from build123d import *

# Parameters (mm, degrees)
SKETCH1_W                = 25
SKETCH1_H                = 120.5
SKETCH1_H_2              = 25
BOSS_EXTRUDE1_DEPTH      = 25
SKETCH1_8_W              = 25
SKETCH1_8_H              = 25
BOSS_EXTRUDE2_DEPTH      = 90
SKETCH1_9_W              = 25
SKETCH1_9_H              = 25
BOSS_EXTRUDE3_DEPTH      = 90
BOSS_EXTRUDE3_DEPTH_BACK = 130
BOSS_EXTRUDE4_DEPTH      = 75
BOSS_EXTRUDE4_DEPTH_BACK = 100
SKETCH3_R                = 16
SKETCH3_R_2              = 12.5
BOSS_EXTRUDE5_DEPTH      = 2
BOSS_EXTRUDE5_DEPTH_BACK = 2
SKETCH4_R                = 16
BOSS_EXTRUDE6_DEPTH      = 2
BOSS_EXTRUDE6_DEPTH_BACK = 2


with BuildPart() as part:
    # Sketch1 → Boss-Extrude1 (new body)
    with BuildSketch(Plane(origin=(0, 0, 0), x_dir=(1, 0, 0), z_dir=(0, 1, 0))):
        with Locations((-72.566666667, -14.316666667)):
            Rectangle(SKETCH1_W, SKETCH1_H)
        with Locations((-72.566666667, 58.433333333)):
            Rectangle(SKETCH1_W, SKETCH1_H_2)
        with Locations((-72.566666667, -87.066666667)):
            Rectangle(SKETCH1_W, SKETCH1_H_2)
    extrude(amount=BOSS_EXTRUDE1_DEPTH)

    # Sketch1_8 → Boss-Extrude2 (add)
    with BuildSketch(Plane(origin=(0, 0, 0), x_dir=(1, 0, 0), z_dir=(0, 1, 0))):
        with Locations((-72.566666667, 58.433333333)):
            Rectangle(SKETCH1_8_W, SKETCH1_8_H)
        with Locations((-72.566666667, -87.066666667)):
            Rectangle(SKETCH1_8_W, SKETCH1_8_H)
    extrude(amount=BOSS_EXTRUDE2_DEPTH)

    # Sketch1_9 → Boss-Extrude3 (add, two sides)
    with BuildSketch(Plane(origin=(0, 0, 0), x_dir=(1, 0, 0), z_dir=(0, 1, 0))) as boss_extrude3_sk:
        with Locations((-72.566666667, -87.066666667)):
            Rectangle(SKETCH1_9_W, SKETCH1_9_H)
    extrude(amount=BOSS_EXTRUDE3_DEPTH)
    extrude(boss_extrude3_sk.sketch, amount=-BOSS_EXTRUDE3_DEPTH_BACK)

    # Sketch2 → Boss-Extrude4 (add, two sides)
    with BuildSketch(Plane(origin=(-60.066666667, 0, 0), x_dir=(0, 0, -1), z_dir=(1, 0, 0))) as boss_extrude4_sk:
        with BuildLine():
            ThreePointArc((-99.566666667, -117.5), (-95.905501431, -126.338834765), (-87.066666667, -130))
            ThreePointArc((-87.066666667, -130), (-82.283123762, -129.048494156), (-78.227831902, -126.338834765))
            Line((-78.227831902, -126.338834765), (-95.905501431, -108.661165235))
            ThreePointArc((-95.905501431, -108.661165235), (-98.615160823, -112.716457095), (-99.566666667, -117.5))
        make_face()
        with BuildLine():
            Line((-95.905501431, -108.661165235), (-78.227831902, -126.338834765))
            ThreePointArc((-78.227831902, -126.338834765), (-75.51817251, -122.283542905), (-74.566666667, -117.5))
            ThreePointArc((-74.566666667, -117.5), (-78.227831902, -108.661165235), (-87.066666667, -105))
            ThreePointArc((-87.066666667, -105), (-91.850209571, -105.951505844), (-95.905501431, -108.661165235))
        make_face()
    extrude(amount=BOSS_EXTRUDE4_DEPTH)
    extrude(boss_extrude4_sk.sketch, amount=-BOSS_EXTRUDE4_DEPTH_BACK)

    # Sketch3 → Boss-Extrude5 (add, two sides)
    with BuildSketch(Plane(origin=(14.933333333, 0, 0), x_dir=(0, 0, -1), z_dir=(1, 0, 0))) as boss_extrude5_sk:
        with Locations((-87.066666667, -117.5)):
            Circle(SKETCH3_R)
        with Locations((-87.066666667, -117.5)):
            Circle(SKETCH3_R_2, mode=Mode.SUBTRACT)
        with BuildLine():
            ThreePointArc((-74.566666667, -117.5), (-78.227831902, -108.661165235), (-87.066666667, -105))
            Line((-87.066666667, -105), (-87.066666667, -130))
            ThreePointArc((-87.066666667, -130), (-78.227831902, -126.338834765), (-74.566666667, -117.5))
        make_face()
        with BuildLine():
            Line((-87.066666667, -130), (-87.066666667, -105))
            ThreePointArc((-87.066666667, -105), (-99.566666667, -117.5), (-87.066666667, -130))
        make_face()
    extrude(amount=BOSS_EXTRUDE5_DEPTH)
    extrude(boss_extrude5_sk.sketch, amount=-BOSS_EXTRUDE5_DEPTH_BACK)

    # Sketch4 → Boss-Extrude6 (add, two sides)
    with BuildSketch(Plane.ZY.offset(160.066666667)) as boss_extrude6_sk:
        with Locations((87.066666667, -117.5)):
            Circle(SKETCH4_R)
    extrude(amount=BOSS_EXTRUDE6_DEPTH)
    extrude(boss_extrude6_sk.sketch, amount=-BOSS_EXTRUDE6_DEPTH_BACK)


solid = part.part
Input: part model. Units: mm. Frame: model coordinates. A direction names the side the tool comes from. Give positions to 0.01 mm unless a question says otherwise; leave off trailing zeros. Order: outer loops, then holes, each group sorted by start corner. A loop starts at its lowest first (then second) coordinate and runs counter-clockwise, first axis right, second up.
Q1. Ray query, probe 1 along Z at (x, y) = (-70, -19); probe 2 along Y at (x, z) = (-60.5, -60); probe 3 along X at (y, z) = (-24, 89.5). Return the intervals inside material, ascending.
Checked values:
probe 1: z = 74.57 to 99.57
probe 2: y = 0 to 90
probe 3: x = -85.07 to -60.07
Q2. Draft query along Z for faces 5 (the flat face through (-73, 57, -45.933)), 6 (the flat face through (-73, 57, 74.567)), 7 (the flat face through (16.933, -117, 87)), 8 (the flat face through (-73, -64, 74.567)). Return one class per face: +Z half, -Z half, draft (parallel to the pull), parting line (faces both ways), or undercut.
Checked values:
face 5: undercut
face 6: undercut
face 7: draft
face 8: -Z half
Q3. Section B-B on x = -64.5. Output: boundary loops of the cut face in (y, z), and give its area (3 significant figures).
Checked values:
outline: (-130, 74.57) - (0, 74.57) - (0, -70.93) - (90, -70.93) - (90, -45.93) - (25, -45.93) - (25, 74.57) - (90, 74.57) - (90, 99.57) - (-130, 99.57) - close
area: 10,800 mm2
Q4. Set-up query: faces 1 (the cylindrical face through (14.961, -112.694, 71.806)), 2 (the flat face through (-85.067, -127, 77)), 3 (the flat face through (-60.067, -127, 97)), 4 (the flat face through (-73, -130, 87)). Return all of +Z, -Z, +X, -X, +Y, -Y with unobstructed straight access to the full face (end or side cutting, diameter ignored); none if empty.
Checked values:
face 1: +X
face 2: -Z, -Y
face 3: +Z, -Y
face 4: +Z, -Z, -Y
Q5. Contact query for flat-ended pins moving along their axis: pin 1 Ø12.5 at (x, z) = (-69.5, 21) entering from -Y; pin 2 Ø20 at (x, y) = (-69.5, 45.5) entering from +Z; pin 3 Ø2 at (x, z) = (-75, 33) entering from +Y. Output: stop coordinate, or through.
Checked values:
pin 1: stops at y = 0
pin 2: stops at z = 99.57
pin 3: stops at y = 25
Q6. Section D-D on y = 3.5. Output: boundary loops of the cut face in (x, z).
Checked values:
outline: (-85.07, -70.93) - (-60.07, -70.93) - (-60.07, 99.57) - (-85.07, 99.57) - close
Q7. Section A-A on y = 56. Output: boundary loops of the cut face in (x, z), and give its area (3 significant figures).
Checked values:
outline: (-85.07, -70.93) - (-60.07, -70.93) - (-60.07, -45.93) - (-85.07, -45.93) - close; (-85.07, 74.57) - (-60.07, 74.57) - (-60.07, 99.57) - (-85.07, 99.57) - close
area: 1,250 mm2
Q8. Section C-C on z = -23.5. Output: boundary loops of the cut face in (x, y).
Checked values:
outline: (-85.07, 0) - (-60.07, 0) - (-60.07, 25) - (-85.07, 25) - close
